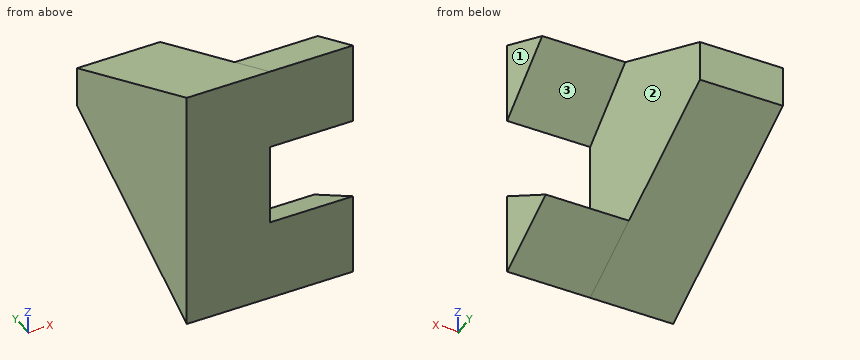
from build123d import *

# Parameters (mm, degrees)
BOSS_EXTRUDE1_DEPTH = 2
BOSS_EXTRUDE2_DEPTH = 2


with BuildPart() as part:
    # Sketch1 → Boss-Extrude1 (new body)
    with BuildSketch(Plane(origin=(0, 0, 0), x_dir=(0, 0, -1), z_dir=(1, 0, 0))):
        Polygon((0, 0), (2.5, 5), (3.5, 5), (6, 0), align=None)
    extrude(amount=BOSS_EXTRUDE1_DEPTH)

    # Sketch2 → Boss-Extrude2 (add)
    with BuildSketch(Plane(origin=(2, 0, 0), x_dir=(0, 0, -1), z_dir=(1, 0, 0))):
        Polygon((0, 0), (2, 0), (0.800710083, 1.601420167), align=None)
        Polygon((4, 0), (6, 0), (5.116370384, 1.767259231), align=None)
    extrude(amount=BOSS_EXTRUDE2_DEPTH)


solid = part.part
Model file for the job. Use its own axes, mm. Face numbers are marked on the shaded views. Coordinates: 2 decimals unless noted, no trailing zeros. Loops run counter-clockwise (first coordinate to the right, second up) from the corner with the lowest first, then second, coordinate; pieces in that order, holes last. Notation, with made-up numbers: (-0.75, 72) -> (13.25, 72) arc R26 cw to (13.25, 87) -> close; hole circle Ø10 at (-35, -35.5). An arc over 180 degrees is marked (long way). Use one line per item in the form item = value. Start each with the question number.
(1) Probe probe 1 along X at (y, z) = (1.8, -3.05); probe 2 along Y at (x, z) = (1.4, -4); probe 3 along Z at (x, y) = (2.2, 0.55) (3 decimals). List the from-to ranges inside material, lowest first. Write a range as from..to.
(2) Flat gauge pins, fed straight in: pin 1 (2 mm diameter, centred on x = 2, z = -4.5, fed in from -Y); pin 2 (3 mm diameter, centred on y = 4.5, z = -4.5, fed in from +X). Where does each tip first touch, or does it go through?
(3) Cut at C-C on z = -5.3. Give the cut face in (x, y).
(4) Cut at B-B on y = 1.5. Give the cut face in (x, z), and give its area (3 significant figures).
(5) Cut at D-D on x = 1.6. Give the cut face in (y, z), and give its area (3 significant figures).
(6) Pull direction Z, two halves, no side cores. Call the marked faces 1, 2 and 3: pulls with the +Z half, pulls with the -Z half, needs draft (parallel to the pull), parting line crosses it, or undercut.
(7) Cut at A-A on x = 2.9. Give the cut face in (y, z).
Values:
q1.probe_1 = 0..2
q1.probe_2 = 0..4
q1.probe_3 = -5.725..-4.347, -1.588..-0.275
q2.pin_1 = 0
q2.pin_2 = 2
q3.outline = (0, 0) -> (4, 0) -> (4, 1.4) -> (0, 1.4) -> close
q4.outline = (0, -5.25) -> (4, -5.25) -> (4, -4.95) -> (2, -4.95) -> (2, -0.88) -> (4, -0.88) -> (4, -0.75) -> (0, -0.75) -> close
q4.area = 9.86 mm2
q5.outline = (0, -6) -> (5, -3.5) -> (5, -2.5) -> (0, 0) -> close
q5.area = 17.5 mm2
q6.face_1 = needs draft
q6.face_2 = undercut
q6.face_3 = undercut
q7.outline = (0, -6) -> (1.77, -5.12) -> (0, -4) -> close; (0, -2) -> (1.6, -0.8) -> (0, 0) -> close
